Input: part model. Units: mm. Frame: model coordinates. A direction names the side the tool comes from. Round coordinates to 2 decimals unless told otherwise and drop trailing zeros. Write each loop counter-clockwise with the first axis right and the second up, starting at its lowest first coordinate (ties: lowest second). Pieces come first, ordered by that corner, then holes. Notation, with made-up numbers: (53, -27.75) -> (66, -27.75) arc R15 cw to (66, -7.75) -> close; hole circle Ø7 at (74, 52.5). An arc over 180 degrees is marked (long way). Use CSV: the item, a comma, the result in double quotes.
```python
from build123d import *

# Parameters (mm, degrees)
PAD002_DEPTH = 102.5
PAD003_DEPTH = 60


with BuildPart() as pad007:
    # Sketch006 → Pad002 (new body, symmetric)
    with BuildSketch(Plane(origin=(0, 0, 0.0001), x_dir=(0, 1, 0), z_dir=(1, 0, 0))):
        with BuildLine():
            ThreePointArc((-42, -13), (-39.87868, -12.12132), (-39, -10))
            Line((-39, -10), (47, -10))
            ThreePointArc((47, -10), (47.87868, -12.12132), (50, -13))
            Line((55, -13), (50, -13))
            Line((55, -33), (55, -13))
            Line((-55, -33), (55, -33))
            Line((-55, -13), (-55, -33))
            Line((-55, -13), (-42, -13))
        make_face()
    extrude(amount=PAD002_DEPTH, both=True)


with BuildPart() as pad008:
    # Sketch005 → Pad003 (new body, symmetric)
    with BuildSketch(Plane.XZ):
        with BuildLine():
            ThreePointArc((-80, -13), (-77.87868, -12.12132), (-77, -10))
            Line((0, -10), (-77, -10))
            Line((0, -32), (0, -10))
            Line((-100, -32), (0, -32))
            Line((-100, -13), (-100, -32))
            Line((-100, -13), (-80, -13))
        make_face()
    extrude(amount=PAD003_DEPTH, both=True)


with BuildPart() as part_mirroring:
    # Part__Mirroring: instance of Pad008
    add(pad008.part.mirror(Plane(origin=(0, 0, 0), x_dir=(0, -1, 0), z_dir=(1, 0, 0))))


with BuildPart() as common:
    # Fusion base: copy of Pad008
    add(pad008.part)

    # Fusion: union Part__Mirroring
    add(part_mirroring.part)

    # Common: intersect Pad007
    add(pad007.part, mode=Mode.INTERSECT)


solid = common.part
```
Item 1: Line query: line 1 (Z direction, x = 58, y = 50.5); line 2 (Y direction, x = 34.5, z = -12.25); line 3 (Y direction, x = 20.5, z = -11.75). Output: solid intervals per line, ascending.
Worked answers:
line 1,"z = -32 to -13"
line 2,"y = -40.02 to 48.02"
line 3,"y = -39.56 to 47.56"
Item 2: Set-up query: faces 1 (the face through (90, -1, -13)), 2 (the face through (1, -49, -13)), 3 (the face through (1, 53, -13)), 4 (the face through (-1, 3, -10)), 5 (the face through (-90, -1, -13)). Return all of +Z, -Z, +X, -X, +Y, -Y with unobstructed straight access to the full face (end or side cutting, diameter ignored); none if empty.
Worked answers:
face 1,"+Z, +X, +Y, -Y"
face 2,"+Z, +X, -X, -Y"
face 3,"+Z, +X, -X, +Y"
face 4,"+Z, +X, -X, +Y, -Y"
face 5,"+Z, -X, +Y, -Y"
Item 3: Section query B-B on y = 9. Return the cut outline in (x, z), plus the area to 3 significant figures.
Worked answers:
outline,"(-100, -32) -> (100, -32) -> (100, -13) -> (80, -13) arc R3 cw to (77, -10) -> (-77, -10) arc R3 cw to (-80, -13) -> (-100, -13) -> close"
area,"4,270 mm²"
Item 4: First-contact query: pin 1 Ø14.5 at (x, y) = (23, -49.5) entering from +Z. Flat tip, straight axial feed; report the tip coordinate or a pass-through.
Worked answers:
pin 1,"stops at z = -13"
Item 5: Section query A-A on x = 56.5. Return the cut outline in (y, z), plus the area to 3 significant figures.
Worked answers:
outline,"(-55, -32) -> (55, -32) -> (55, -13) -> (50, -13) arc R3 cw to (47, -10) -> (-39, -10) arc R3 cw to (-42, -13) -> (-55, -13) -> close"
area,"2,350 mm²"
